Could you check a few things on this model? Use its own coordinates, in mm. A direction names the side the tool comes from. Coordinates: 2 decimals unless noted, no trailing zeros. Order: outer loops, then holes, each group sorted by start corner. A loop starts at its lowest first (then second) coordinate and runs counter-clockwise, first axis right, second up.
```python
from build123d import *

# Parameters (mm, degrees)
BOSS_EXTRUDE1_DEPTH     = 16
CUT_EXTRUDE1_DEPTH      = 15
SKETCH3_R               = 1.002930515
SKETCH3_W               = 12.5
SKETCH3_H               = 1
CUT_EXTRUDE2_DEPTH      = 11
SKETCH4_W               = 3
SKETCH4_H               = 1.5
CUT_EXTRUDE3_DEPTH      = 1
CUT_EXTRUDE3_DEPTH_BACK = 44
SKETCH5_R               = 1
SKETCH5_R_2             = 0.75
CUT_EXTRUDE4_DEPTH      = 1


with BuildPart() as part:
    # Sketch1 → Boss-Extrude1 (new body)
    with BuildSketch(Plane(origin=(0, 0, 0), x_dir=(1, 0, 0), z_dir=(0, 1, 0))):
        Polygon((-21.5, 15.276990566), (-15.910083809, 21), (15.910083809, 21), (21.5, 15.276990566), (21.5, -15.276990566), (15.910083809, -21), (-15.910083809, -21), (-21.5, -15.276990566), align=None)
    extrude(amount=BOSS_EXTRUDE1_DEPTH)

    # Sketch2 → Cut-Extrude1 (cut)
    with BuildSketch(Plane(origin=(0, 16, 0), x_dir=(1, 0, 0), z_dir=(0, 1, 0))):
        Polygon((-15.488962048, 20), (-20.5, 14.869651621), (-20.5, -14.869651621), (-15.488962048, -20), (15.488962048, -20), (20.5, -14.869651621), (20.5, 14.869651621), (15.488962048, 20), align=None)
    extrude(amount=-CUT_EXTRUDE1_DEPTH, mode=Mode.SUBTRACT)

    # Sketch3 → Cut-Extrude2 (cut)
    with BuildSketch(Plane(origin=(0, 16, 0), x_dir=(1, 0, 0), z_dir=(0, 1, 0))):
        with Locations((16.5, 12.271619794)):
            Circle(SKETCH3_R)
        with Locations((7.988962048, 20.5)):
            Rectangle(SKETCH3_W, SKETCH3_H)
    extrude(amount=-CUT_EXTRUDE2_DEPTH, mode=Mode.SUBTRACT)

    # Sketch4 → Cut-Extrude3 (cut, two sides)
    with BuildSketch(Plane.ZY.offset(21.5)) as cut_extrude3_sk:
        with Locations((-11.369651621, 12.25)):
            Rectangle(SKETCH4_W, SKETCH4_H)
        with Locations((11.369651621, 12.25)):
            Rectangle(SKETCH4_W, SKETCH4_H)
    extrude(amount=CUT_EXTRUDE3_DEPTH, mode=Mode.SUBTRACT)
    extrude(cut_extrude3_sk.sketch, amount=-CUT_EXTRUDE3_DEPTH_BACK, mode=Mode.SUBTRACT)

    # Sketch5 → Cut-Extrude4 (cut)
    with BuildSketch(Plane(origin=(0, 1, 0), x_dir=(1, 0, 0), z_dir=(0, 1, 0))):
        with Locations((16, 13)):
            Circle(SKETCH5_R)
        with Locations((8.5, 17)):
            Circle(SKETCH5_R_2)
    extrude(amount=-CUT_EXTRUDE4_DEPTH, mode=Mode.SUBTRACT)


solid = part.part
```
Item 1: For pin 1 Ø2 at (x, z) = (8.5, -17) entering from +Y; pin 2 Ø0.5 at (x, y) = (21, 12.5) entering from +Z; pin 3 Ø0.5 at (x, y) = (-21, 12) entering from -Z, each with a flat end and sliding along its axis, tell me the tip position at first contact or that it passes through.
Item 2: Suppose I cut it at D-D (z = -17). List the corners of the cut face in (x, y) for me, and give its area (3 significant figures).
Item 3: I need wall thicknesses on line 1 (Z direction, x = 8.5, y = 0.75); line 2 (X direction, y = 0.35, z = -13); line 3 (Z direction, x = -12.5, y = 4). Which ranges of each line are inside material? Lowest first, please.
Item 4: Suppose I cut it at B-B (y = 2.5). List the corners of the cut face in (x, z) for me.
Item 5: Suppose I cut it at C-C (x = 0.5). List the corners of the cut face in (y, z) for me, and give its area (3 significant figures).
Item 6: Which directions (+Z, -Z, +X, -X, +Y, -Y) give clear straight access to the entire face, cutting with the end or side of a thin tool? Please do faces 3 (the face through (0, 9, 20)), 4 (the face through (7.905, 0.507, -16.544)), 5 (the face through (21, 12, 12.87)).
Item 7: Thinking about a two-plate mould opening in Y: for faces 1 (the face through (-21, 12, -9.87)), 2 (the face through (-21.5, 8, 0)), which applies, +Y half, -Y half, draft (parallel to the pull), parting line (faces both ways), or undercut?
Item 8: Suppose I cut it at A-A (x = 8.5). List the corners of the cut face in (y, z) for me.
Geometry results:
1. pin 1: stops at y = 1
1. pin 2: stops at z = 16.04
1. pin 3: stops at z = -16.04
2. outline: (-19.82, 0) - (7.75, 0) - (7.75, 1) - (-18.42, 1) - (-18.42, 16) - (-19.82, 16) - close; (9.25, 0) - (19.82, 0) - (19.82, 16) - (18.42, 16) - (18.42, 1) - (9.25, 1) - close
2. area: 80.1 mm2
3. line 1: z = -21 to -17.75, -16.25 to 21
3. line 2: x = -21.5 to 15, 17 to 21.5
3. line 3: z = -21 to -20, 20 to 21
4. outline: (-21.5, -15.28) - (-15.91, -21) - (15.91, -21) - (21.5, -15.28) - (21.5, 15.28) - (15.91, 21) - (-15.91, 21) - (-21.5, 15.28) - close; hole (-20.5, -14.87) - (-15.49, -20) - (15.49, -20) - (20.5, -14.87) - (20.5, 14.87) - (15.49, 20) - (-15.49, 20) - (-20.5, 14.87) - close
5. outline: (0, -21) - (16, -21) - (16, -20) - (1, -20) - (1, 20) - (16, 20) - (16, 21) - (0, 21) - close
5. area: 72.0 mm2
6. face 3: +Y
6. face 4: +Y, -Y
6. face 5: +X, -X
7. face 1: undercut
7. face 2: draft
8. outline: (0, -21) - (5, -21) - (5, -20) - (1, -20) - (1, -17.75) - (0, -17.75) - close; (0, -16.25) - (1, -16.25) - (1, 20) - (16, 20) - (16, 21) - (0, 21) - close
